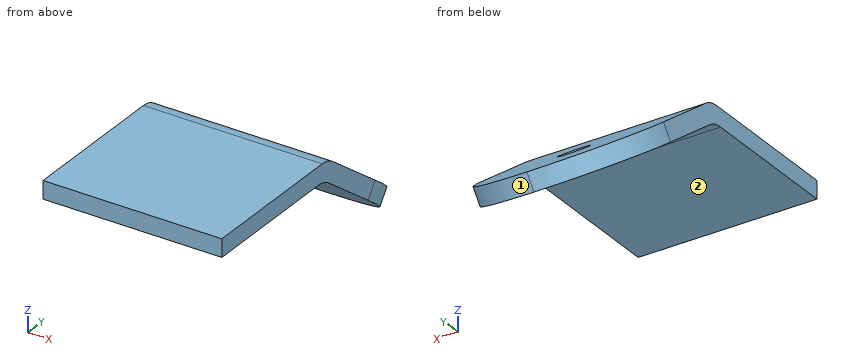
```python
from build123d import *

# Parameters (mm, degrees)
F1_DEPTH = 10
F3_D     = 3.3
F4_R     = 3
F5_R     = 9.99999


# Not quite as in the source:
# - a fillet or chamfer is up to 0.001 mm smaller than in the source, because OpenCascade refuses the exact size


with BuildPart() as f1:
    # F0 (on Right) → F1 (new body, symmetric)
    with BuildSketch(Plane.YZ):
        Polygon((-8.9946911595, 33.2547011177), (-26.9946911595, 33.2547011177), (-26.9946911595, 31.2547011177), (-9.6638817985, 31.2547011177), (5.7743889952, 19.6211296345), (6.9780190415, 21.2184006546), align=None)
    extrude(amount=F1_DEPTH, both=True)

    # F3 (through all)
    with Locations(Plane(origin=(0, 12.7255260612, 16.8873434619), x_dir=(1, 0, 0), z_dir=(0, 0.6018150232, 0.79863551))):
        with Locations((0, -17.1966584849)):
            Hole(F3_D / 2)

    # F4
    f4_edges = [f1.edges().sort_by_distance(p)[0] for p in [
        (0, -8.994691, 33.254701),
        (0, -9.663882, 31.254701),
    ]]
    fillet(f4_edges, radius=F4_R)

    # F5 (radius 10 in the source; OpenCascade refuses exactly that, so slightly less here)
    f5_edges = [f1.edges().sort_by_distance(p)[0] for p in [
        (10, 6.376204, 20.419765),
        (-10, 6.376204, 20.419765),
    ]]
    fillet(f5_edges, radius=F5_R)


solid = f1.part
```
Build history of the part. All positions in model axes, mm. Face numbers are marked on the shaded views. A direction names the side the tool comes from. Round coordinates to 2 decimals unless told otherwise and drop trailing zeros. Write each loop counter-clockwise with the first axis right and the second up, starting at its lowest first coordinate (ties: lowest second). Pieces come first, ordered by that corner, then holes. Notation, with made-up numbers: (57.5, -34) - (104.5, -34) arc R20 ccw to (104.5, -17) - close; hole circle Ø6 at (2, 61). An arc over 180 degrees is marked (long way). Write each question's results on one line, items separated by ' | '. Start each with the question number.
Item 1: Saw through at C-C (x = 7.25). Write the cut outline in (y, z).
Item 2: Saw through at B-B (y = -23). Write the cut outline in (x, z).
Item 3: Wall check: L1, parallel to Z at x = 5.25, y = -14.5; L2, parallel to Y at x = 5.75, z = 29.5; L3, parallel to Y at x = -8, z = 28. Give the ranges that are in metal, low to high. Write a range as [from, to].
Item 4: Which spindle directions (+Z, -Z, +X, -X, +Y, -Y) get a long thin tool onto all of the face, cutting with end or side? Do the marked faces 1 and 2. Say none if no direction does.
Item 5: Drop flat-ended pins along their axis: P1, Ø8, axis at x = -4.5, y = -22, coming from the -Z side; P2, Ø4, axis at x = 2.5, y = 0.5, coming from the -Z side; P3, Ø6, axis at x = 2.5, y = 0.5, coming from the +Z side. Give the stop position or say it passes through.
Item 6: Saw through at D-D (z = 30). Write the cut outline in (x, y).
Item 7: Saw through at A-A (x = 1.25). Write the cut outline in (y, z), and give its area (3 significant figures).
Results are:
1) outline: (-26.99, 31.25) - (-10.67, 31.25) arc R3 cw to (-8.86, 30.65) - (3.29, 21.49) - (4.49, 23.09) - (-8.19, 32.65) arc R3 ccw to (-10, 33.25) - (-26.99, 33.25) - close
2) outline: (-10, 31.25) - (10, 31.25) - (10, 33.25) - (-10, 33.25) - close
3) L1: z = [31.25, 33.25] | L2: y = [-7.34, -4.01] | L3: y = [-5.34, -2.02]
4) face 1: -Z, +X, +Y | face 2: -Z, +X, -X, -Y
5) P1: stops at z = 31.25 | P2: stops at z = 22.09 | P3: stops at z = 28.36
6) outline: (-10, -8) - (10, -8) - (10, -4.68) - (-10, -4.68) - close
7) outline: (-26.99, 31.25) - (-10.67, 31.25) arc R3 cw to (-8.86, 30.65) - (-3.07, 26.29) - (-1.87, 27.88) - (-8.19, 32.65) arc R3 ccw to (-10, 33.25) - (-26.99, 33.25) - close; (-1.35, 24.99) - (5.71, 19.67) - (6.92, 21.27) - (-0.15, 26.59) - close | area: 70.2 mm²
